```python
from build123d import *

# Parameters (mm, degrees)
SKETCH1_W           = 400
SKETCH1_H           = 210
SKETCH1_W_2         = 394
SKETCH1_H_2         = 204
EXTRUDE_THIN1_DEPTH = 250
SKETCH4_R           = 25
CUT_EXTRUDE1_DEPTH  = 10


with BuildPart() as part:
    # Sketch1 → Extrude-Thin1 (new body)
    with BuildSketch(Plane(origin=(0, 0, 0), x_dir=(1, 0, 0), z_dir=(0, 1, 0))):
        with Locations((200, -105)):
            Rectangle(SKETCH1_W, SKETCH1_H)
        with Locations((200, -105)):
            Rectangle(SKETCH1_W_2, SKETCH1_H_2, mode=Mode.SUBTRACT)
    extrude(amount=EXTRUDE_THIN1_DEPTH)

    # Sketch4 → Cut-Extrude1 (cut)
    with BuildSketch(Plane(origin=(0, 0, 0), x_dir=(-1, 0, 0), z_dir=(0, 0, -1))):
        with Locations((-300, 200)):
            Circle(SKETCH4_R)
    extrude(amount=-CUT_EXTRUDE1_DEPTH, mode=Mode.SUBTRACT)


solid = part.part
```
The model under review builds one solid part; all positions refer to its coordinate system, in mm. A direction names the side the tool comes from. Give positions to 0.01 mm unless a question says otherwise; leave off trailing zeros. Order: outer loops, then holes, each group sorted by start corner. A loop starts at its lowest first (then second) coordinate and runs counter-clockwise, first axis right, second up. Notation, with made-up numbers: (32, -32) - (62, -32) arc R16 cw to (62, -2) - close; hole circle Ø3 at (6, -34.5). An arc over 180 degrees is marked (long way). Use CSV: the item, a comma, the result in double quotes. Start each with the question number.
Q1. We need section A-A, the plane z = 22. Write out the cut boundary in (x, y).
Q2. To check wall thickness, follow line 1 along Z through (x, y) = (201, 201.5); line 2 along X through (y, z) = (63, 29); line 3 along Y through (x, z) = (300, 1). State the ranges of each line that lie inside material, in increasing order. Write a range as [from, to].
Q3. We need section C-C, the plane y = 200. Write out the cut boundary in (x, z).
Q4. The part is to be moulded in two halves that separate along Z. For faces 3 (the flat face through (197, 123, 0)), 4 (the flat face through (197, 123, 3)), 5 (the cylindrical face through (276.154, 207.509, 1.479)), say which applies: +Z half, -Z half, draft (parallel to the pull), parting line (faces both ways), or undercut.
Q5. Clearance check with a flat-ended pin moving along its axis: pin 1 Ø4 at (y, z) = (176, 148.5) entering from -X. State where the tip first meets the part, or that it passes through.
Q6. We need section B-B, the plane x = 300. Write out the cut boundary in (y, z).
Q7. Tool access review of faces 1 (the flat face through (197, 123, 207)), 2 (the flat face through (197, 123, 210)): name each direction out of +Z, -Z, +X, -X, +Y, -Y from which nothing blocks a thin tool from reaching the whole face with its end or side.
Q8. We need section D-D, the plane x = 240.5. Write out the cut boundary in (y, z).
Outcome:
1,outline,"(0, 0) - (3, 0) - (3, 250) - (0, 250) - close; (397, 0) - (400, 0) - (400, 250) - (397, 250) - close"
2,line 1,"z = [0, 3], [207, 210]"
2,line 2,"x = [0, 3], [397, 400]"
2,line 3,"y = [0, 175], [225, 250]"
3,outline,"(0, 0) - (275, 0) - (275, 3) - (3, 3) - (3, 207) - (397, 207) - (397, 3) - (325, 3) - (325, 0) - (400, 0) - (400, 210) - (0, 210) - close"
4,face 3,"-Z half"
4,face 4,"undercut"
4,face 5,"draft"
5,pin 1,"stops at x = 0"
6,outline,"(0, 0) - (175, 0) - (175, 3) - (0, 3) - close; (0, 207) - (250, 207) - (250, 210) - (0, 210) - close; (225, 0) - (250, 0) - (250, 3) - (225, 3) - close"
7,face 1,"+Y, -Y"
7,face 2,"+Z, +X, -X, +Y, -Y"
8,outline,"(0, 0) - (250, 0) - (250, 3) - (0, 3) - close; (0, 207) - (250, 207) - (250, 210) - (0, 210) - close"
